Verification items for this drawing (mm, ordinates from the low corner). A direction names the side the tool comes from. Give positions to 0.01 mm unless a question says otherwise; leave off trailing zeros. Write each loop counter-clockwise with the first axis right and the second up, starting at its lowest first coordinate (ties: lowest second). Pieces come first, ordered by that corner, then holes. Notation, with made-up numbers: (0.5, 84.5) -> (35.5, 84.5) arc R21 cw to (35.5, 120.5) -> close; hole circle Ø2 at (83, 87.5). An arc over 180 degrees is marked (long way). Answer as a JSON object with one key per item and string values.
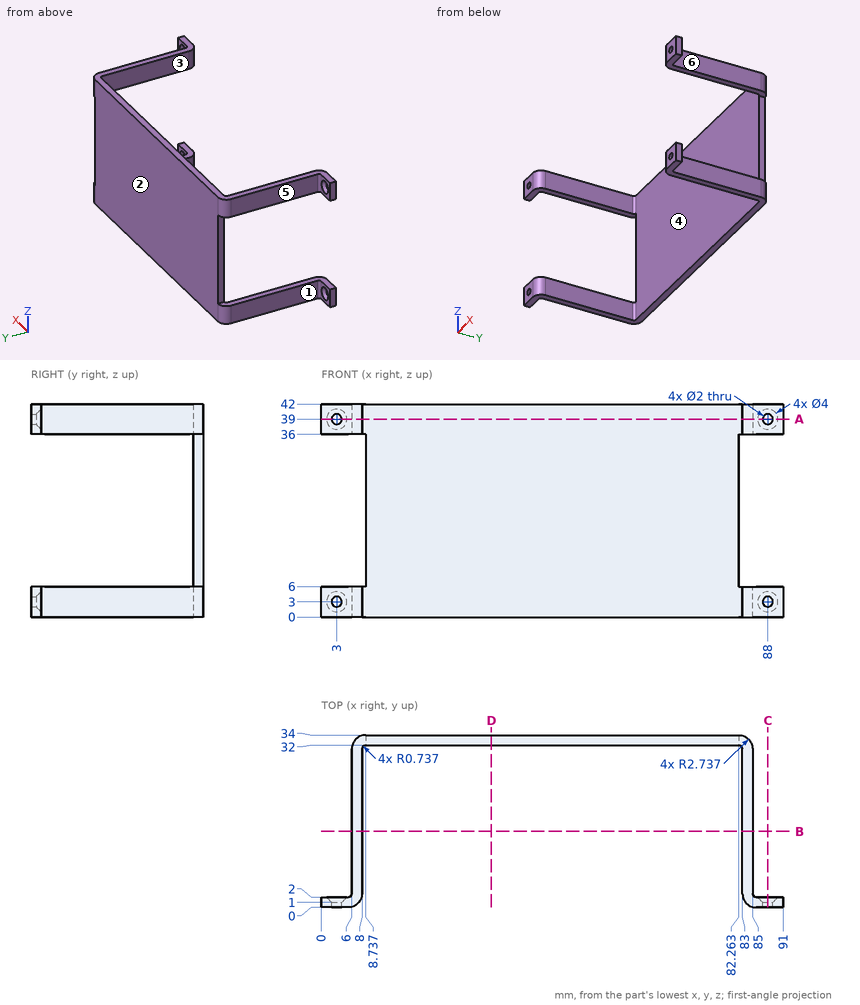
1. Go/stop test with flat-tipped pins: P1, Ø4, axis at x = 3.5, z = 2, coming from the +Y side; P2, Ø3, axis at y = 21.5, z = 3, coming from the -X side; P3, Ø2, axis at y = 7.5, z = 6.5, coming from the +X side; P4, Ø4.5, axis at x = 88, y = 15, coming from the -Z side (1 decimal). Record where each tip stops, or that it passes through.
Determined:
{"P1": "y = 2.04", "P2": "x = 6", "P3": "x = 85", "P4": "through"}
2. Sectioned sample at C-C, the plane x = 88. Enter the section's corners in (y, z).
Determined:
{"outline": "(0, 0) -> (2, 0) -> (2, 1) -> (1, 2) -> (0, 2) -> close; (0, 4) -> (1, 4) -> (2, 5) -> (2, 6) -> (0, 6) -> close; (0, 36) -> (2, 36) -> (2, 37) -> (1, 38) -> (0, 38) -> close; (0, 40) -> (1, 40) -> (2, 41) -> (2, 42) -> (0, 42) -> close"}
3. Sectioned sample at D-D, the plane x = 33.5. Enter the section's corners in (y, z).
Determined:
{"outline": "(32, 0) -> (34, 0) -> (34, 42) -> (32, 42) -> close"}
4. Mould release check, pull along X, two halves, no side actions. Record for the marked faces 1, 2 and 3: released by +X, released by -X, zero draft, split by the parting line, or undercut.
Determined:
{"face 1": "released by -X", "face 2": "zero draft", "face 3": "undercut"}
5. Sectioned sample at A-A, the plane z = 39. State how many separate pieces and enclosed holes the cut face has, plus the area to 3 significant figures.
Determined:
{"separate pieces": "3", "enclosed holes": "0", "area": "294 mm^2"}
6. Access from +Z, -Z, +X, -X, +Y, -Y to the whole of each face (thin tool, end or side, straight path). Record for the marked faces 4, 5 and 6.
Determined:
{"face 4": "+Z, -Z, -Y", "face 5": "+Z, -Z, -X, +Y", "face 6": "+Z, -Z, +X, +Y"}
7. Scan lines: L1, parallel to Z at x = 88, y = 0.45; L2, parallel to X at y = 0.35, z = 39 (1 decimal); L3, parallel to Y at x = 28, z = 20.5. Record each from-to range of solid material in increasing order. Write a range as [from, to].
Determined:
{"L1": "[0, 2], [4, 6], [36, 38], [40, 42]", "L2": "[0, 2], [4, 6.6], [84.4, 87], [89, 91]", "L3": "[32, 34]"}
8. Sectioned sample at B-B, the plane y = 15. Enter the section's corners in (x, z).
Determined:
{"outline": "(6, 0) -> (8, 0) -> (8, 6) -> (6, 6) -> close; (6, 36) -> (8, 36) -> (8, 42) -> (6, 42) -> close; (83, 0) -> (85, 0) -> (85, 6) -> (83, 6) -> close; (83, 36) -> (85, 36) -> (85, 42) -> (83, 42) -> close"}
